CAD build for the part. Positions are in the model's coordinates, mm. Give positions to 0.01 mm unless a question says otherwise; leave off trailing zeros. Write each loop counter-clockwise with the first axis right and the second up, starting at its lowest first coordinate (ties: lowest second). Pieces come first, ordered by that corner, then holes. Notation, with made-up numbers: (54.5, 29) - (88.5, 29) arc R35 cw to (88.5, 63) - close; hole circle Ø10 at (87.5, 40). An arc over 180 degrees is marked (long way). Put each result on its own line as item: value. Start each with the question number.
1. Wall check: line 1 (Y direction, x = 145.5, z = 3.15); line 2 (Y direction, x = -126, z = 3.8); line 3 (Y direction, x = 25.5, z = 2.75). Give the ranges that are in metal, low to high.
2. Cut at D-D on z = 3. Give the number of separate pieces and of enclosed holes in the cut face, and give its area (3 significant figures).
3. Cut at A-A on y = -85. List the corners of the cut face in (x, z), and give its area (3 significant figures).
4. Cut at C-C on x = 120.5. List the corners of the cut face in (y, z).
5. Drop flat-ended pins along their axis: pin 1 (2.5 mm diameter, centred on x = -100.46, y = -102.52, fed in from +Z); pin 2 (1.5 mm diameter, centred on x = -67, z = 3, fed in from +Y); pin 3 (1.8 mm diameter, centred on y = -202.5, z = 2, fed in from -X); pin 4 (1.1 mm diameter, centred on y = 2, z = 1.5, fed in from +X). Give the stop position or say it passes through.
6. Cut at B-B on x = -5. List the corners of the cut face in (y, z), and give its area (3 significant figures).
7. Mould opens along Y. For faces 1 (the cylindrical face through (-2.405, -70.255, 1.972)), 2 (the flat face through (-30, -99, 0)) say: +Y half, -Y half, draft (parallel to the pull), parting line (faces both ways), or undercut.
from build123d import *

# Parameters (mm, degrees)
SKETCH_1_R          = 1.5
SKETCH_1_R_2        = 30
SKETCH_1_W          = 4.4
SKETCH_1_H          = 8.4
EXTRUDE_1_DEPTH     = 4
SKETCH_4_R          = 1.5
CUT_EXTRUDE_1_DEPTH = 10
FILLET_1_R          = 1.3


with BuildPart() as part:
    # 草图1 → 凸台-拉伸1 (new body)
    with BuildSketch(Plane.XY):
        Polygon((0, 0), (0, -4), (-1.35, -4), (-1.35, -6.6), (0, -6.6), (0, -8.6), (3, -8.6), (3, -6.6), (4.35, -6.6), (4.35, -4), (3, -4), (3, 0), (30.5, 0), (30.5, 5), (38.5, 5), (38.5, 0), (66, 0), (66, -4), (64.65, -4), (64.65, -6.6), (66, -6.6), (66, -8.6), (69, -8.6), (69, -6.6), (70.35, -6.6), (70.35, -4), (69, -4), (69, 0), (96.5, 0), (96.5, 5), (104.5, 5), (104.5, 0), (132, 0), (143.5, 0), (145.5, 0), (150.5, 0), (150.5, -200), (145.5, -200), (143.5, -200), (132, -200), (104.5, -200), (104.5, -205), (96.5, -205), (96.5, -200), (69, -200), (69, -196), (70.35, -196), (70.35, -193.4), (69, -193.4), (69, -191.4), (66, -191.4), (66, -193.4), (64.65, -193.4), (64.65, -196), (66, -196), (66, -200), (38.5, -200), (38.5, -205), (30.5, -205), (30.5, -200), (3, -200), (3, -196), (4.35, -196), (4.35, -193.4), (3, -193.4), (3, -191.4), (0, -191.4), (0, -193.4), (-1.35, -193.4), (-1.35, -196), (0, -196), (0, -200), (-27.5, -200), (-27.5, -205), (-35.5, -205), (-35.5, -200), (-63, -200), (-63, -196), (-61.65, -196), (-61.65, -193.4), (-63, -193.4), (-63, -191.4), (-66, -191.4), (-66, -193.4), (-67.35, -193.4), (-67.35, -196), (-66, -196), (-66, -200), (-93.5, -200), (-93.5, -205), (-101.5, -205), (-101.5, -200), (-129, -200), (-140.5, -200), (-142.5, -200), (-147.5, -200), (-147.5, 0), (-142.5, 0), (-140.5, 0), (-129, 0), (-101.5, 0), (-101.5, 5), (-93.5, 5), (-93.5, 0), (-66, 0), (-66, -4), (-67.35, -4), (-67.35, -6.6), (-66, -6.6), (-66, -8.6), (-63, -8.6), (-63, -6.6), (-61.65, -6.6), (-61.65, -4), (-63, -4), (-63, 0), (-35.5, 0), (-35.5, 5), (-27.5, 5), (-27.5, 0), align=None)
        with Locations((-142.5, -100)):
            Circle(SKETCH_1_R, mode=Mode.SUBTRACT)
        with Locations(Location((145.5, -100, 0), (0, 0, 180))):
            Circle(SKETCH_1_R, mode=Mode.SUBTRACT)
        with Locations((1.5, -100)):
            Circle(SKETCH_1_R_2, mode=Mode.SUBTRACT)
        with Locations((-142.5, -67)):
            Rectangle(SKETCH_1_W, SKETCH_1_H, mode=Mode.SUBTRACT)
        with Locations((-142.5, -133)):
            Rectangle(SKETCH_1_W, SKETCH_1_H, mode=Mode.SUBTRACT)
        with Locations((145.5, -133)):
            Rectangle(SKETCH_1_W, SKETCH_1_H, mode=Mode.SUBTRACT)
        with Locations((145.5, -67)):
            Rectangle(SKETCH_1_W, SKETCH_1_H, mode=Mode.SUBTRACT)
    extrude(amount=EXTRUDE_1_DEPTH)

    # 草图4 → 切除-拉伸1 (cut)
    with BuildSketch(Plane.XY.offset(4)):
        with Locations((-100.464854909, -102.524202067)):
            Circle(SKETCH_4_R)
        with Locations((-72.564854909, -102.524202067)):
            Circle(SKETCH_4_R)
        with Locations((-112.964854909, -153.324202067)):
            Circle(SKETCH_4_R)
        with Locations((-67.464854909, -154.624202067)):
            Circle(SKETCH_4_R)
        with Locations((-117.464854909, -35.441983185)):
            Circle(SKETCH_4_R)
        with Locations((-68.464854909, -35.441983185)):
            Circle(SKETCH_4_R)
        with Locations((-117.464854909, -93.441983185)):
            Circle(SKETCH_4_R)
        with Locations((-68.464854909, -93.441983185)):
            Circle(SKETCH_4_R)
    extrude(amount=-CUT_EXTRUDE_1_DEPTH, mode=Mode.SUBTRACT)

    # 圆角1
    fillet_1_edges = [part.edges().sort_by_distance(p)[0] for p in [
        (30.5, 5, 2),
        (38.5, 5, 2),
        (96.5, 5, 2),
        (104.5, 5, 2),
        (104.5, -205, 2),
        (96.5, -205, 2),
        (38.5, -205, 2),
        (30.5, -205, 2),
        (-27.5, -205, 2),
        (-35.5, -205, 2),
        (-93.5, -205, 2),
        (-101.5, -205, 2),
        (-101.5, 5, 2),
        (-93.5, 5, 2),
        (-35.5, 5, 2),
        (-27.5, 5, 2),
    ]]
    fillet(fillet_1_edges, radius=FILLET_1_R)


solid = part.part
Report:
1. line 1: y = -200 to -137.2, -128.8 to -101.5, -98.5 to -71.2, -62.8 to 0
1. line 2: y = -200 to 0
1. line 3: y = -200 to -118, -82 to 0
2. separate pieces: 1
2. enclosed holes: 15
2. area: 56,700 mm²
3. outline: (-147.5, 0) - (-24.48, 0) - (-24.48, 4) - (-147.5, 4) - close; (27.48, 0) - (150.5, 0) - (150.5, 4) - (27.48, 4) - close
3. area: 984 mm²
4. outline: (-200, 0) - (0, 0) - (0, 4) - (-200, 4) - close
5. pin 1: passes through
5. pin 2: stops at y = 0
5. pin 3: stops at x = -101.5
5. pin 4: stops at x = 104.5
6. outline: (-200, 0) - (-129.29, 0) - (-129.29, 4) - (-200, 4) - close; (-70.71, 0) - (0, 0) - (0, 4) - (-70.71, 4) - close
6. area: 566 mm²
7. face 1: undercut
7. face 2: draft
